Part print with two shaded views. Sizes in mm from the minimum x, y, z corner. A direction names the side the tool comes from. Give positions to 0.01 mm unless a question says otherwise; leave off trailing zeros. Order: outer loops, then holes, each group sorted by start corner. A loop starts at its lowest first (then second) coordinate and runs counter-clockwise, first axis right, second up. Notation, with made-up numbers: (37.5, -5.75) - (41.5, -5.75) arc R22 ccw to (41.5, 18.25) - close; hole circle Ø7 at (29, 41.25). An arc over 180 degrees is marked (long way). Return JSON: item names as keys, results as strings. Group by question number.
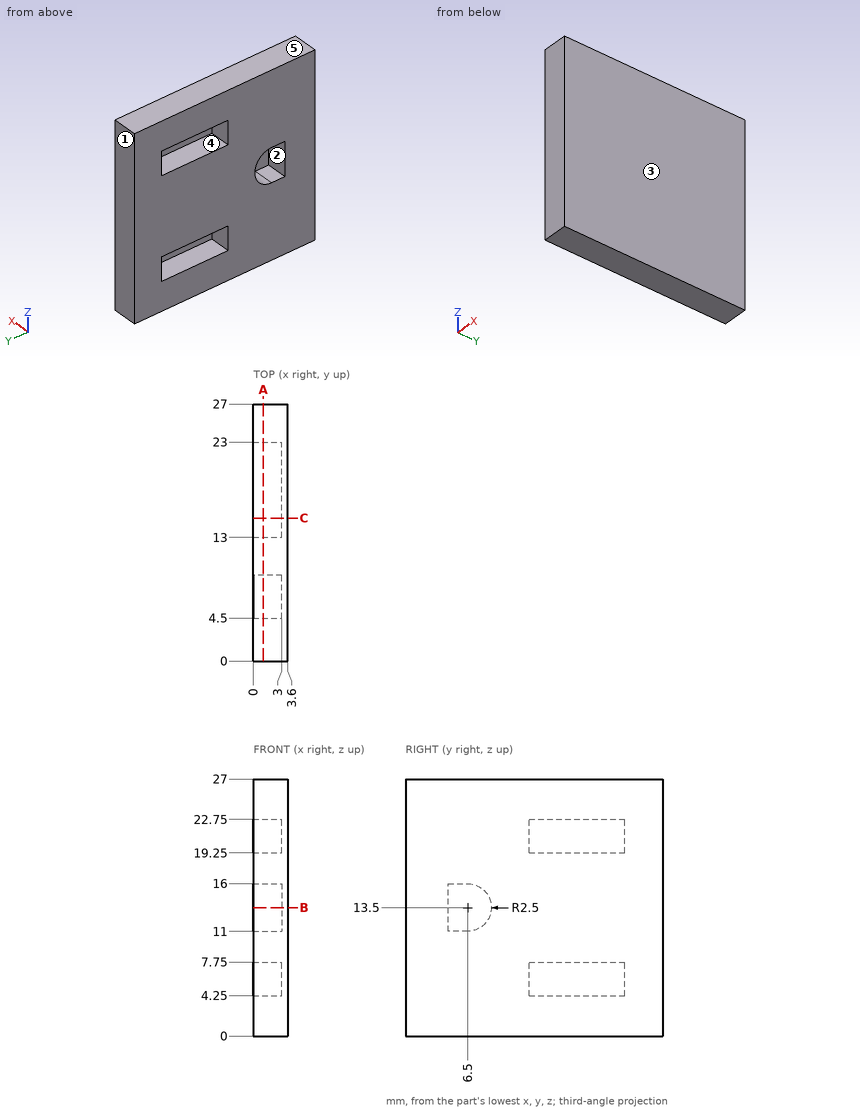
(1) Slice it at C-C (y = 15). Give the cut face in (x, z).
(2) Drop a flat-ended pin along its axis: pin 1 Ø1 at (y, z) = (16.5, 6) entering from -X. Give the stop position or say it passes through.
(3) 3-axis set-ups, long thin cutter, end or side, ignore diameter. For the marked faces 4 and 5: which of +Z, -Z, +X, -X, +Y, -Y reach the whole face in a straight line?
(4) Pull direction Y, two halves, no side cores. Call the marked faces 1, 2 and 3: released by +Y, released by -Y, zero draft, split by the parting line, or undercut.
(5) Slice it at A-A (x = 1.05). Give the cut face in (y, z), and give its area (3 significant figures).
(6) Slice it at B-B (z = 13.5). Give the cut face in (x, y), and give its area (3 significant figures).
(7) Drill centre lines: L1, parallel to Z at x = 2.05, y = 20; L2, parallel to Z at x = 2.5, y = 5.5; L3, parallel to Y at x = 2.55, z = 19.5. Where is each one in solid material? Low to high.
Result set:
{
 "1": {"outline": "(0, 0) - (3.6, 0) - (3.6, 27) - (0, 27) - (0, 22.75) - (3, 22.75) - (3, 19.25) - (0, 19.25) - (0, 7.75) - (3, 7.75) - (3, 4.25) - (0, 4.25) - close"},
 "2": {"pin 1": "stops at x = 3"},
 "3": {"face 4": "-X", "face 5": "+Z, +X, -X, +Y, -Y"},
 "4": {"face 1": "released by +Y", "face 2": "undercut", "face 3": "zero draft"},
 "5": {"outline": "(0, 0) - (27, 0) - (27, 27) - (0, 27) - close; hole (4.5, 11) - (6.5, 11) arc R2.5 ccw to (6.5, 16) - (4.5, 16) - close; hole (13, 4.25) - (23, 4.25) - (23, 7.75) - (13, 7.75) - close; hole (13, 19.25) - (23, 19.25) - (23, 22.75) - (13, 22.75) - close", "area": "639 mm²"},
 "6": {"outline": "(0, 0) - (3.6, 0) - (3.6, 27) - (0, 27) - (0, 9) - (3, 9) - (3, 4.5) - (0, 4.5) - close", "area": "83.7 mm²"},
 "7": {"L1": "z = 0 to 4.25, 7.75 to 19.25, 22.75 to 27", "L2": "z = 0 to 11, 16 to 27", "L3": "y = 0 to 13, 23 to 27"}
}
